Source: CAD feature listing. Evaluate the final solid. Frame: model axes, mm. Coordinates: 2 decimals unless noted, no trailing zeros. Write each loop counter-clockwise with the first axis right and the second up, starting at its lowest first coordinate (ties: lowest second). Pieces come first, ordered by that corner, then holes. Notation, with made-up numbers: (81, 3.5) - (87, 3.5) arc R25 cw to (87, 39.5) - close; hole circle Ø9 at (40, 36.5). An arc over 180 degrees is marked (long way). One line per question, with ' | ' between items.
from build123d import *

# Parameters (mm, degrees)
BOSS_EXTRUDE1_DEPTH             = 3.175
F_1_2_0_5_DIAMETER_HOLE1_D      = 12.7
F_5_16_0_3125_DIAMETER_HOLE1_D  = 7.9375
F_5_32_0_15625_DIAMETER_HOLE1_D = 3.96875
F_7_64_0_10938_DIAMETER_HOLE1_D = 2.778252
F_6_CLEARANCE_HOLE1_D           = 4.3053


with BuildPart() as part:
    # Sketch1 → Boss-Extrude1 (new body)
    with BuildSketch(Plane.XY):
        with BuildLine():
            Line((157.767651581, 0), (1.5875, 0))
            ThreePointArc((1.5875, 0), (0.464967985, -0.464967985), (0, -1.5875))
            Line((0, -1.5875), (0, -23.8125))
            ThreePointArc((0, -23.8125), (0.464967985, -24.935032015), (1.5875, -25.4))
            Line((1.5875, -25.4), (163.5125, -25.4))
            ThreePointArc((163.5125, -25.4), (164.635032015, -24.935032015), (165.1, -23.8125))
            Line((165.1, -23.8125), (165.1, -11.537869343))
            ThreePointArc((165.1, -11.537869343), (165.045907249, -11.126994109), (164.887315329, -10.744119343))
            Line((164.887315329, -10.744119343), (159.14246691, -0.79375))
            ThreePointArc((159.14246691, -0.79375), (158.561401581, -0.212684671), (157.767651581, 0))
        make_face()
    extrude(amount=BOSS_EXTRUDE1_DEPTH)

    # 1/2 (0.5) Diameter Hole1 (through all)
    with Locations(Plane(origin=(0, 0, 0), x_dir=(-1, 0, 0), z_dir=(0, 0, -1))):
        with Locations((-53.975, -10.16), (-88.9, -10.16)):
            Hole(F_1_2_0_5_DIAMETER_HOLE1_D / 2)

    # 5/16 (0.3125) Diameter Hole1 (through all)
    with Locations(Plane(origin=(0, 0, 0), x_dir=(-1, 0, 0), z_dir=(0, 0, -1))):
        with Locations((-14.2875, -11.43)):
            Hole(F_5_16_0_3125_DIAMETER_HOLE1_D / 2)

    # 5/32 (0.15625) Diameter Hole1 (through all)
    with Locations(Plane(origin=(0, 0, 0), x_dir=(-1, 0, 0), z_dir=(0, 0, -1))):
        with Locations((-21.598282462, -11.43)):
            Hole(F_5_32_0_15625_DIAMETER_HOLE1_D / 2)

    # 7/64 (0.10938) Diameter Hole1 (through all)
    with Locations(Plane(origin=(0, 0, 0), x_dir=(-1, 0, 0), z_dir=(0, 0, -1))):
        with Locations((-88.959471598, -19.537541197), (-63.423407807, -10.16)):
            Hole(F_7_64_0_10938_DIAMETER_HOLE1_D / 2)

    # #6 Clearance Hole1 (through all)
    with Locations(Plane(origin=(0, 0, 0), x_dir=(-1, 0, 0), z_dir=(0, 0, -1))):
        with Locations((-158.75, -18.415), (-117.475, -8.89), (-30.48, -16.51)):
            Hole(F_6_CLEARANCE_HOLE1_D / 2)


solid = part.part
Item 1: Cut plane A-A on x = 30.48. Return loops of the section in (y, z) (3 decimals), and give its area (3 significant figures).
Check sheet entries:
outline: (-25.4, 0) - (-18.663, 0) - (-18.663, 3.175) - (-25.4, 3.175) - close; (-14.357, 0) - (0, 0) - (0, 3.175) - (-14.357, 3.175) - close | area: 67.0 mm²
Item 2: Ray query, line 1 along Y through (x, z) = (88.9, 2.4); line 2 along Y through (x, z) = (30.48, 2.3); line 3 along X through (y, z) = (-8, 2.55). Return the intervals inside material, ascending. Write a range as [from, to].
Check sheet entries:
line 1: [-25.4, -20.93], [-18.15, -16.51], [-3.81, 0] | line 2: [-25.4, -18.66], [-14.36, 0] | line 3: [0, 12.29], [16.28, 48], [59.95, 82.93], [94.87, 115.51], [119.44, 163.3]
Item 3: Mould query, pull axis Y, two halves, no side actions, for faces 1 (the face through (88.78, -18.16, 1.61)), 2 (the face through (81, -13, 0)), 3 (the face through (162.055, -5.839, 1.565)). Classes: pulls with the +Y half, pulls with the -Y half, needs draft (parallel to the pull), parting line crosses it, or undercut.
Check sheet entries:
face 1: undercut | face 2: needs draft | face 3: pulls with the +Y half
Item 4: Pin query (flat end, axial travel): pin 1 Ø2.5 at (x, y) = (21.6, -11.43) entering from -Z. Return the tip coordinate at first contact, or that it passes through.
Check sheet entries:
pin 1: through
Item 5: Cut plane B-B on z = 2.6. State how many separate pieces and enclosed holes the cut face has, and give its area (3 significant figures).
Check sheet entries:
separate pieces: 1 | enclosed holes: 9 | area: 3,790 mm²
